Work out the finished part from the listing and answer in its coordinate system (mm). A direction names the side the tool comes from. Coordinates: 2 decimals unless noted, no trailing zeros. Order: outer loops, then holes, each group sorted by start corner. A loop starts at its lowest first (then second) coordinate and runs counter-clockwise, first axis right, second up.
```python
from build123d import *

# Parameters (mm, degrees)
BOSS_EXTRUDE1_DEPTH = 25.4
FILLET1_R           = 2.54


with BuildPart() as part:
    # Sketch1 → Boss-Extrude1 (new body)
    with BuildSketch(Plane(origin=(0, 0, 0), x_dir=(1, 0, 0), z_dir=(0, 1, 0))):
        with BuildLine():
            Line((-244.848924974, -184.847069368), (-240.047965661, -181.222617027))
            ThreePointArc((-240.047965661, -181.222617027), (-245.557867235, -173.683610566), (-250.831084415, -165.977196721))
            Line((-250.831084415, -165.977196721), (-255.847706103, -169.296740655))
            ThreePointArc((-255.847706103, -169.296740655), (-250.469024579, -177.157282777), (-244.848924974, -184.847069368))
        make_face()
        with BuildLine():
            ThreePointArc((-215.750093665, -209.562782535), (-228.339131483, -195.770027771), (-240.047965661, -181.222617027))
            Line((-240.047965661, -181.222617027), (-244.848924974, -184.847069368))
            ThreePointArc((-244.848924974, -184.847069368), (-238.99238799, -192.359230601), (-232.905461186, -199.685956603))
            ThreePointArc((-232.905461186, -199.685956603), (-226.594481496, -206.819670414), (-220.065095538, -213.754038186))
            Line((-220.065095538, -213.754038186), (-215.750093665, -209.562782535))
        make_face()
        with BuildLine():
            ThreePointArc((-232.905461186, -199.685956603), (-238.99238799, -192.359230601), (-244.848924974, -184.847069368))
            Line((-244.848924974, -184.847069368), (-260.051962799, -196.32450178))
            ThreePointArc((-260.051962799, -196.32450178), (-254.20265496, -203.841466748), (-248.136139057, -211.184255684))
            Line((-248.136139057, -211.184255684), (-232.905461186, -199.685956603))
        make_face()
    extrude(amount=BOSS_EXTRUDE1_DEPTH)

    # Fillet1
    fillet1_edges = [part.edges().sort_by_distance(p)[0] for p in [
        (-220.065095538, 12.7, 213.754038186),
        (-248.136139057, 12.7, 211.184255684),
        (-260.051962799, 12.7, 196.32450178),
        (-255.847706103, 12.7, 169.296740655),
    ]]
    fillet(fillet1_edges, radius=FILLET1_R)


solid = part.part
```
1. The part is cut by section B-B (z = 205). Determine the outline of the cut face in (x, y), plus the area to 3 significant figures.
2. The part is cut by section D-D (z = 176.5). Determine the outline of the cut face in (x, y).
3. For faces 1 (the flat face through (-242, 0, 194)), 2 (the flat face through (-251.341, 12.522, 189.748)), 3 (the cylindrical face through (-227.53, 12.52, 205.79)), determine the directions among +Z, -Z, +X, -X, +Y, -Y from which every point of the face is accessible in a straight line to the end or side of a thin tool.
4. The mould has two halves that part along Z. Classify faces 4 (the cylindrical face through (-254.804, 12.878, 169.484)), 5 (the cylindrical face through (-259, 12.88, 196.45)), 6 (the cylindrical face through (-254.22, 12.52, 203.82)), 7 (the cylindrical face through (-249.8, 12.5, 178.1)): released by +Z, released by -Z, zero draft, split by the parting line, or undercut.
5. The part is cut by section A-A (y = 17.5). Determine the outline of the cut face in (x, z).
6. The part is cut by section C-C (x = -220.5). Determine the outline of the cut face in (y, z), plus the area to 3 significant figures.
7. Consider probe 1 along X at (y, z) = (20.5, 202.5); probe 2 along X at (y, z) = (22, 205); probe 3 along X at (y, z) = (5, 195). Determine where each line is inside the solid, lowest interval first.
8. Flat-ended cylindrical pins translate along their axes: pin 1 (10 mm diameter, centred on x = -241.5, y = 18, fed in from -Z); pin 2 (8 mm diameter, centred on y = 9.5, z = 177.5, fed in from +X); pin 3 (1.5 mm diameter, centred on y = 11.5, z = 188, fed in from +X). Find the tip coordinate at first contact, or state that the pin passes through.
Worked out:
1. outline: (-253.27, 0) - (-239.94, 0) - (-239.94, 25.4) - (-253.27, 25.4) - close; (-228.24, 0) - (-220.09, 0) - (-220.09, 25.4) - (-228.24, 25.4) - close
1. area: 546 mm2
2. outline: (-250.93, 0) - (-243.54, 0) - (-243.54, 25.4) - (-250.93, 25.4) - close
3. face 1: +Z, -Z, +X, -X, -Y
3. face 2: -X, +Y, -Y
3. face 3: +Z, +Y, -Y
4. face 4: undercut
4. face 5: split by the parting line
4. face 6: released by +Z
4. face 7: undercut
5. outline: (-258.5, 198.36) arc R2.54 ccw to (-258.02, 194.79) - (-244.85, 184.85) arc R306.79 ccw to (-254.43, 171.43) arc R2.54 ccw to (-253.72, 167.89) - (-250.83, 165.98) arc R300.77 cw to (-215.75, 209.56) - (-218.24, 211.98) arc R2.54 ccw to (-221.84, 211.91) arc R306.79 ccw to (-232.91, 199.69) - (-246.22, 209.74) arc R2.54 ccw to (-249.69, 209.34) arc R325.84 ccw to start
6. outline: (0, 204.56) - (25.4, 204.56) - (25.4, 212.65) - (0, 212.65) - close
6. area: 205 mm2
7. probe 1: x = -255.27 to -236.63, -230.46 to -222.39
7. probe 2: x = -253.27 to -239.94, -228.24 to -220.09
7. probe 3: x = -258.26 to -229
8. pin 1: stops at z = 172.34
8. pin 2: stops at x = -239.84
8. pin 3: stops at x = -234.18
